Can you work these out from the drawing? Everything is in mm from the part's minimum corner. Round coordinates to 2 decimals unless told otherwise and drop trailing zeros. Write each loop counter-clockwise with the first axis right and the second up, starting at its lowest first coordinate (ties: lowest second). Pieces come first, ordered by that corner, then holes. Notation, with made-up numbers: M -16,89 L -1,89 A19 ccw -1,98 Z; hole C 37,63.5 d11. An arc over 180 degrees is marked long. Use one line per item in the form item = value. Start each with the question number.
Q1. I want a section at A-A on x = 10. List the corners of the cut face in (y, z) for me (1 decimal).
Q2. I want a section at B-B on z = 31.75. List the corners of the cut face in (x, y) for me (1 decimal).
Q3. I need wall thicknesses on line 1 along Z through (x, y) = (10, 2.05); line 2 along X through (y, z) = (0.4, 19.5). Which ranges of each line are inside material? Lowest first, please. Write a range as from..to.
Q4. I want a section at D-D on x = 27. List the corners of the cut face in (y, z) for me (1 decimal).
Q5. I want a section at C-C on z = 53.5. List the corners of the cut face in (x, y) for me (1 decimal), and give its area (3 significant figures).
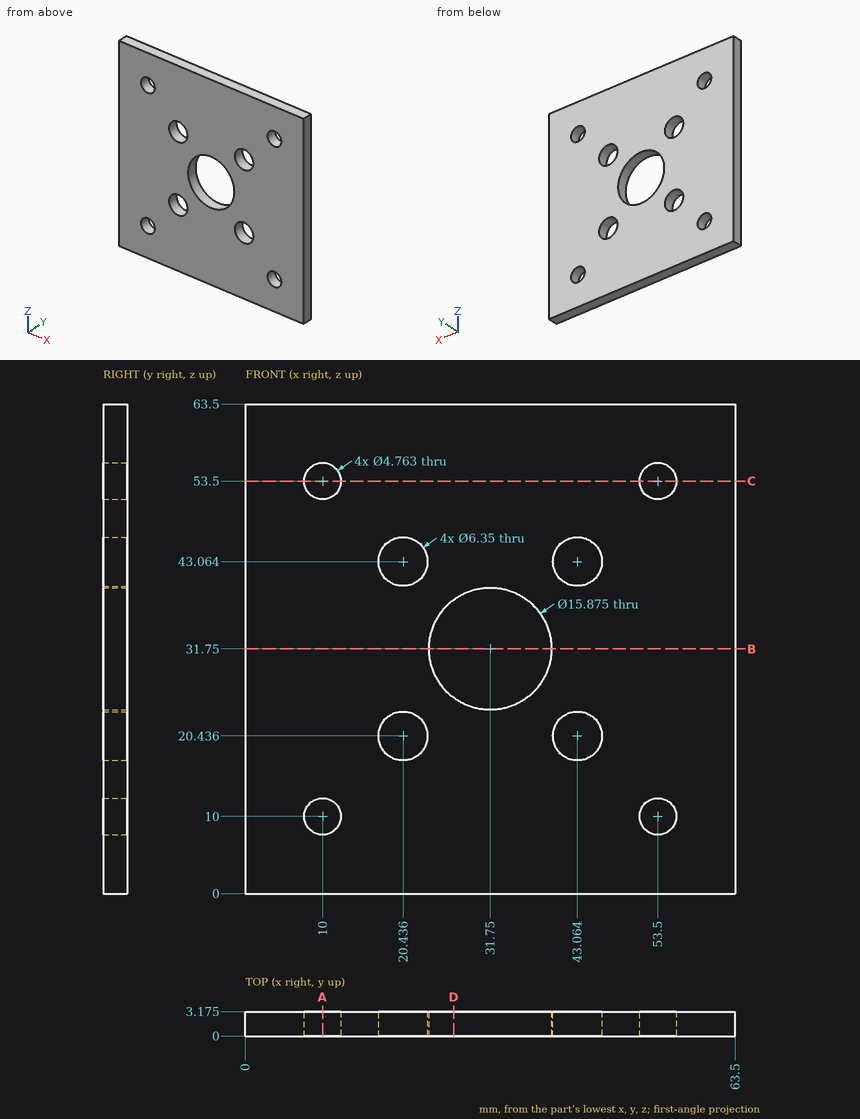
Reported:
q1.outline = M 0,0 L 3.2,0 L 3.2,7.6 L 0,7.6 Z; M 0,12.4 L 3.2,12.4 L 3.2,51.1 L 0,51.1 Z; M 0,55.9 L 3.2,55.9 L 3.2,63.5 L 0,63.5 Z
q2.outline = M 0,0 L 23.8,0 L 23.8,3.2 L 0,3.2 Z; M 39.7,0 L 63.5,0 L 63.5,3.2 L 39.7,3.2 Z
q3.line_1 = 0..7.62, 12.38..51.12, 55.88..63.5
q3.line_2 = 0..17.4, 23.47..40.03, 46.1..63.5
q4.outline = M 0,0 L 3.2,0 L 3.2,25.4 L 0,25.4 Z; M 0,38.1 L 3.2,38.1 L 3.2,63.5 L 0,63.5 Z
q5.outline = M 0,0 L 7.6,0 L 7.6,3.2 L 0,3.2 Z; M 12.4,0 L 51.1,0 L 51.1,3.2 L 12.4,3.2 Z; M 55.9,0 L 63.5,0 L 63.5,3.2 L 55.9,3.2 Z
q5.area = 171 mm^2
